Can you work these out from the model? Positions are in its coordinate system, mm. Face numbers are marked on the shaded views. A direction names the side the tool comes from. Give positions to 0.01 mm unless a question says otherwise; leave off trailing zeros. Order: outer loops, then holes, each group sorted by start corner. A loop starts at its lowest first (then second) coordinate and runs counter-clockwise, first axis right, second up. Notation, with made-up numbers: (-16.5, 73.25) - (34.5, 73.25) arc R32 cw to (34.5, 112.25) - close; hole circle Ø4 at (65.5, -40). An arc over 180 degrees is marked (long way). One line per question, with ' | ' between items.
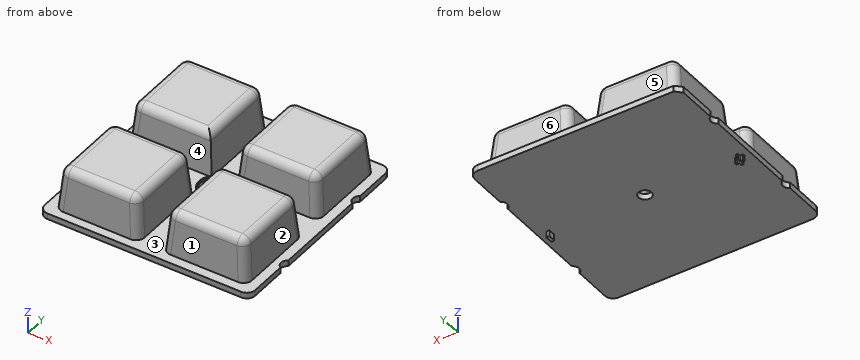
```python
from build123d import *

# Parameters (mm, degrees)
F0_R     = 1.55
F1_DEPTH = 1.4
F2_W     = 20
F2_H     = 20
F3_DEPTH = 10
F3_TAPER = 5
F4_R     = 3.75
F4_R_2   = 3.5
F5_DEPTH = 0.5
F7_DEPTH = 1.4
F8_R     = 2


with BuildPart() as f1:
    # F0 (on Top) → F1 (new body)
    with BuildSketch(Plane.XY):
        with BuildLine():
            Line((23, 25), (-23.5878064872, 25))
            Line((-23.5878064872, 25), (-25, 23.5878064872))
            Line((-25, 23.5878064872), (-25, 14.0856406461))
            ThreePointArc((-25, 14.0856406461), (-24.2, 12.7), (-25, 11.3143593539))
            Line((-25, 11.3143593539), (-25, -11.3143593539))
            ThreePointArc((-25, -11.3143593539), (-24.2, -12.7), (-25, -14.0856406461))
            Line((-25, -14.0856406461), (-25, -23))
            ThreePointArc((-25, -23), (-24.4142135624, -24.4142135624), (-23, -25))
            Line((-23, -25), (23, -25))
            ThreePointArc((23, -25), (24.4142135624, -24.4142135624), (25, -23))
            Line((25, -23), (25, -14.0856406461))
            ThreePointArc((25, -14.0856406461), (24.2, -12.7), (25, -11.3143593539))
            Line((25, -11.3143593539), (25, 11.3143593539))
            ThreePointArc((25, 11.3143593539), (24.2, 12.7), (25, 14.0856406461))
            Line((25, 14.0856406461), (25, 23))
            ThreePointArc((25, 23), (24.4142135624, 24.4142135624), (23, 25))
        make_face()
        Circle(F0_R, mode=Mode.SUBTRACT)
    extrude(amount=F1_DEPTH)

    # F2 (on face) → F3 (join)
    with BuildSketch(Plane.XY.offset(1.4)):
        with Locations((-12.7, 12.8739687322)):
            Rectangle(F2_W, F2_H)
        with Locations((12.6994042229, 12.7)):
            Rectangle(F2_W, F2_H)
        with Locations((12.6994042229, -12.7)):
            Rectangle(F2_W, F2_H)
        with Locations((-12.7, -12.8739687322)):
            Rectangle(F2_W, F2_H)
    extrude(amount=F3_DEPTH, taper=F3_TAPER)

    # F4 (on face) → F5 (join)
    with BuildSketch(Plane.XY.offset(1.4)):
        Circle(F4_R)
        Circle(F4_R_2, mode=Mode.SUBTRACT)
    extrude(amount=F5_DEPTH)

    # F6 (on face) → F7 (join)
    with BuildSketch(Plane(origin=(0, 0, 0), x_dir=(1, 0, 0), z_dir=(0, 0, -1))):
        with BuildLine():
            Line((-22.8843539953, 0.25), (-23.4682458366, 0.25))
            ThreePointArc((-23.4682458366, 0.25), (-23.5, 0), (-23.4682458366, -0.25))
            Line((-23.4682458366, -0.25), (-22.8843539953, -0.25))
            ThreePointArc((-22.8843539953, -0.25), (-22.7951967548, -0.2895183078), (-22.75, -0.3759356876))
            ThreePointArc((-22.75, -0.3759356876), (-22.7484251347, -0.397465641), (-22.75, -0.4189955944))
            Line((-22.75, -0.4189955944), (-22.75, -0.9682458366))
            ThreePointArc((-22.75, -0.9682458366), (-22.5, -1), (-22.25, -0.9682458366))
            Line((-22.25, -0.9682458366), (-22.25, -0.4189955944))
            ThreePointArc((-22.25, -0.4189955944), (-22.2515748653, -0.397465641), (-22.25, -0.3759356876))
            ThreePointArc((-22.25, -0.3759356876), (-22.2048032452, -0.2895183078), (-22.1156460047, -0.25))
            Line((-22.1156460047, -0.25), (-21.5317541634, -0.25))
            ThreePointArc((-21.5317541634, -0.25), (-21.5, 0), (-21.5317541634, 0.25))
            Line((-21.5317541634, 0.25), (-22.1156460047, 0.25))
            ThreePointArc((-22.1156460047, 0.25), (-22.2048032452, 0.2895183078), (-22.25, 0.3759356876))
            ThreePointArc((-22.25, 0.3759356876), (-22.2515748653, 0.397465641), (-22.25, 0.4189955944))
            Line((-22.25, 0.4189955944), (-22.25, 0.9682458366))
            ThreePointArc((-22.25, 0.9682458366), (-22.5, 1), (-22.75, 0.9682458366))
            Line((-22.75, 0.9682458366), (-22.75, 0.4189955944))
            ThreePointArc((-22.75, 0.4189955944), (-22.7484251347, 0.397465641), (-22.75, 0.3759356876))
            ThreePointArc((-22.75, 0.3759356876), (-22.7951967548, 0.2895183078), (-22.8843539953, 0.25))
        make_face()
        with BuildLine():
            Line((-22.75, 0.4189955944), (-22.75, 0.3759356876))
            ThreePointArc((-22.75, 0.3759356876), (-22.7484251347, 0.397465641), (-22.75, 0.4189955944))
        make_face()
        with BuildLine():
            ThreePointArc((-22.75, -0.4189955944), (-22.7484251347, -0.397465641), (-22.75, -0.3759356876))
            Line((-22.75, -0.3759356876), (-22.75, -0.4189955944))
        make_face()
        with BuildLine():
            Line((-22.25, 0.3759356876), (-22.25, 0.4189955944))
            ThreePointArc((-22.25, 0.4189955944), (-22.2515748653, 0.397465641), (-22.25, 0.3759356876))
        make_face()
        with BuildLine():
            ThreePointArc((-22.25, -0.3759356876), (-22.2515748653, -0.397465641), (-22.25, -0.4189955944))
            Line((-22.25, -0.4189955944), (-22.25, -0.3759356876))
        make_face()
        with BuildLine():
            Line((22.1181050964, 0.8344019427), (22.1181050964, -0.8344019427))
            ThreePointArc((22.1181050964, -0.8344019427), (22.5036541776, -0.9220035064), (22.8818949036, -0.8068684502))
            Line((22.8818949036, -0.8068684502), (22.8818949036, 0.8068684502))
            ThreePointArc((22.8818949036, 0.8068684502), (22.5036541776, 0.9220035064), (22.1181050964, 0.8344019427))
        make_face()
    extrude(amount=F7_DEPTH)

    # F8
    f8_edges = [f1.edges().sort_by_distance(p)[0] for p in [
        (-3.574887, 12.873969, 11.4),
        (-12.7, 21.999082, 11.4),
        (-21.825113, 12.873969, 11.4),
        (-12.7, 3.748855, 11.4),
        (12.699404, 3.574887, 11.4),
        (21.824518, 12.7, 11.4),
        (12.699404, 21.825113, 11.4),
        (3.574291, 12.7, 11.4),
        (12.699404, -21.825113, 11.4),
        (21.824518, -12.7, 11.4),
        (12.699404, -3.574887, 11.4),
        (3.574291, -12.7, 11.4),
        (-12.7, -3.748855, 11.4),
        (-21.825113, -12.873969, 11.4),
        (-12.7, -21.999082, 11.4),
        (-3.574887, -12.873969, 11.4),
        (-22.262557, 3.311412, 6.4),
        (-22.262557, -3.311412, 6.4),
        (-22.262557, -22.436525, 6.4),
        (-3.137443, -22.436525, 6.4),
        (3.136848, -22.262557, 6.4),
        (22.261961, -22.262557, 6.4),
        (3.136848, 3.137443, 6.4),
        (22.261961, 3.137443, 6.4),
        (22.261961, 22.262557, 6.4),
        (3.136848, 22.262557, 6.4),
        (-3.137443, 22.436525, 6.4),
        (-22.262557, 22.436525, 6.4),
        (22.261961, -3.137443, 6.4),
        (3.136848, -3.137443, 6.4),
        (-3.137443, -3.311412, 6.4),
    ]]
    fillet(f8_edges, radius=F8_R)


solid = f1.part
```
(1) Imagine slicing it at B-B (y = -18). List the corners of the cut face in (x, z) for me.
Answer below:
outline: (-25, 0) - (25, 0) - (25, 1.4) - (22.7, 1.4) - (21.98, 9.57) arc R2 ccw to (19.99, 11.4) - (5.41, 11.4) arc R2 ccw to (3.41, 9.57) - (2.7, 1.4) - (-2.7, 1.4) - (-3.42, 9.57) arc R2 ccw to (-5.41, 11.4) - (-19.99, 11.4) arc R2 ccw to (-21.98, 9.57) - (-22.7, 1.4) - (-25, 1.4) - close
(2) If I drill on line 1 (Y direction, x = 0, z = 1.65); line 2 (Z direction, x = 6, y = -14.5); line 3 (Y direction, x = 0, z = 0.8), over which ranges is the centre line in solid material (lowest first)?
Answer below:
line 1: -3.75 to -3.5, 3.5 to 3.75 | line 2: 0 to 11.4 | line 3: -25 to -1.55, 1.55 to 25
(3) Imagine slicing it at D-D (z = 3.75). Count the separate pieces of the cut face and the enclosed holes in it, and give its area (3 significant figures).
Answer below:
separate pieces: 4 | enclosed holes: 0 | area: 1,520 mm^2
(4) On a 3-axis mill with a long thin cutter (end or side, diameter ignored), from which of +Z, -Z, +X, -X, +Y, -Y can I reach the whole of each face in a straight line? I mean the marked faces 4, 5 and 6. Say none if no direction works.
Answer below:
face 4: +Z, -X | face 5: +Z, +X, -X, +Y | face 6: +Z, +X, +Y
(5) Will these pins go through, and if not, where does the flat tip stop? pin 1 (1.5 mm diameter, centred on y = 0, z = -1, fed in from +X); pin 2 (1 mm diameter, centred on x = -12, y = -20, fed in from -Z); pin 3 (0.6 mm diameter, centred on x = -23, z = -0.5, fed in from -Y).
Answer below:
pin 1: x = 22.88 | pin 2: z = 0 | pin 3: y = -0.98
(6) Imagine slicing it at C-C (x = -13). List the corners of the cut face in (y, z) for me, and give its area (3 significant figures).
Answer below:
outline: (-25, 0) - (25, 0) - (25, 1.4) - (22.87, 1.4) - (22.16, 9.57) arc R2 ccw to (20.17, 11.4) - (5.58, 11.4) arc R2 ccw to (3.59, 9.57) - (2.87, 1.4) - (-2.87, 1.4) - (-3.59, 9.57) arc R2 ccw to (-5.58, 11.4) - (-20.17, 11.4) arc R2 ccw to (-22.16, 9.57) - (-22.87, 1.4) - (-25, 1.4) - close | area: 450 mm^2
(7) Imagine slicing it at A-A (x = 0). List the corners of the cut face in (y, z) for me.
Answer below:
outline: (-25, 0) - (-1.55, 0) - (-1.55, 1.4) - (-3.5, 1.4) - (-3.5, 1.9) - (-3.75, 1.9) - (-3.75, 1.4) - (-25, 1.4) - close; (1.55, 0) - (25, 0) - (25, 1.4) - (3.75, 1.4) - (3.75, 1.9) - (3.5, 1.9) - (3.5, 1.4) - (1.55, 1.4) - close
(8) If we mould it in two halves opening along X, with no side actions, what happens to the marked faces 1, 2 and 3? For each: released by +X, released by -X, zero draft, split by the parting line, or undercut.
Answer below:
face 1: zero draft | face 2: released by +X | face 3: undercut
